from build123d import *

# Parameters (mm, degrees)
SKETCH_2_OUTSIDE_W  = 16.154
SKETCH_2_OUTSIDE_H  = 16.154
CUT_EXTRUDE_1_DEPTH = 6.2


with BuildPart() as part:
    # Эскиз1 → Повернуть1 (revolve)
    with BuildSketch(Plane.XY):
        Polygon((2.6, 3), (-2.6, 3), (-2.6, 4.5), (-2.051517244, 5.45), (2.051517244, 5.45), (2.6, 4.5), align=None)
    revolve(axis=Axis((-345.378129483, 0, 0), (1, 0, 0)))

    # Эскиз2 outside → Вырез-Вытянуть1 (cut, through all)
    with BuildSketch(Plane.ZY.offset(2.6)):
        Rectangle(SKETCH_2_OUTSIDE_W, SKETCH_2_OUTSIDE_H)
        Polygon((0, -5.773502692), (5, -2.886751346), (5, 2.886751346), (0, 5.773502692), (-5, 2.886751346), (-5, -2.886751346), align=None, mode=Mode.SUBTRACT)
    extrude(amount=-CUT_EXTRUDE_1_DEPTH, mode=Mode.SUBTRACT)


solid = part.part
Check sheet for the modelled part. Datum: model origin and axes. Units: mm. Round coordinates to 2 decimals unless told otherwise and drop trailing zeros. Order: outer loops, then holes, each group sorted by start corner. A loop starts at its lowest first (then second) coordinate and runs counter-clockwise, first axis right, second up.
(1) Go/stop test with flat-tipped pins: P1, Ø1.5, axis at x = 0, z = 3.5, coming from the +Y side; P2, Ø5.5, axis at y = 0, z = 0, coming from the +X side. Record where each tip stops, or that it passes through.
(2) Scan lines: probe 1 along Z at (x, y) = (1.5, -1.5); probe 2 along Z at (x, y) = (0.65, 0); probe 3 along Y at (x, z) = (1.15, -2.5). Record each from-to range of solid material in increasing order.
(3) Draft check along Y on faces 1 (the cylindrical face through (0.029, -2.717, 4.724)), 2 (the flat face through (-0.032, 4.315, 2.526)), 3 (the cylindrical face through (0, -3, 0)), 4 (the flat face through (2.6, 1, -3)). Enter one of: pulls with the +Y half, pulls with the -Y half, needs draft (parallel to the pull), parting line crosses it, or undercut.
(4) Cross-section at B-B, the plane x = -1.35. Enter the section's corners in (y, z), and give its area (3 significant figures).
(5) Cross-section at C-C, the plane y = 0. Enter the section's corners in (x, z), and give its area (3 significant figures).
(6) Cross-section at A-A, the plane z = 0. Enter the section's corners in (x, y), and give its area (3 significant figures).
Check sheet entries:
1. P1: stops at y = 4.19
1. P2: passes through
2. probe 1: z = -5 to -2.6, 2.6 to 5
2. probe 2: z = -5 to -3, 3 to 5
2. probe 3: y = -4.33 to -1.66, 1.66 to 4.33
3. face 1: pulls with the -Y half
3. face 2: pulls with the +Y half
3. face 3: undercut
3. face 4: needs draft
4. outline: (-5.41, -0.62) - (-3.25, -4.38) arc R5.45 ccw to (-2.17, -5) - (2.17, -5) arc R5.45 ccw to (3.25, -4.38) - (5.41, -0.62) arc R5.45 ccw to (5.41, 0.62) - (3.25, 4.38) arc R5.45 ccw to (2.17, 5) - (-2.17, 5) arc R5.45 ccw to (-3.25, 4.38) - (-5.41, 0.62) arc R5.45 ccw to start; hole circle Ø6 at (0, 0)
4. area: 57.2 mm2
5. outline: (-2.6, -4.5) - (-2.31, -5) - (2.31, -5) - (2.6, -4.5) - (2.6, -3) - (-2.6, -3) - close; (-2.6, 3) - (2.6, 3) - (2.6, 4.5) - (2.31, 5) - (-2.31, 5) - (-2.6, 4.5) - close
5. area: 20.5 mm2
6. outline: (-2.6, -4.5) - (-2.05, -5.45) - (2.05, -5.45) - (2.6, -4.5) - (2.6, -3) - (-2.6, -3) - close; (-2.6, 3) - (2.6, 3) - (2.6, 4.5) - (2.05, 5.45) - (-2.05, 5.45) - (-2.6, 4.5) - close
6. area: 24.4 mm2
